Input: part model. Units: mm. Frame: model coordinates. A direction names the side the tool comes from. Give positions to 0.01 mm unless a question says otherwise; leave off trailing zeros. Order: outer loops, then holes, each group sorted by start corner. A loop starts at its lowest first (then second) coordinate and runs counter-clockwise, first axis right, second up. Notation, with made-up numbers: (86, 78) - (98, 78) arc R17 cw to (98, 86) - close; hole circle Ø8 at (4, 22.25). An arc over 180 degrees is marked (long way). Answer in a Markdown table with one row per item. Add a question column.
1. Access query for faces 5 (the face through (0, 213, 101)), 6 (the face through (-1, 79, 100)). Directions: +Z, -Z, +X, -X, +Y, -Y. A direction counts if a zero-diameter tool reaches every point of the face in a straight line with its end or side. Return the directions, or none.
2. Section query D-D on x = -27.5. Return loops of the section in (y, z), and give its area (3 significant figures).
3. Section query A-A on z = 15. Return loops of the section in (x, y), and give its area (3 significant figures).
4. Section query B-B on y = 91.5. Return loops of the section in (x, z), and give its area (3 significant figures).
5. Mould query, pull axis X, two halves, no side actions, for faces 1 (the face through (1, 78, 103)), 2 (the face through (50, 108, 51)), 3 (the face through (-50, 108, 49)), 4 (the face through (-53, 108, 52)). Classes: released by +X, released by -X, zero draft, split by the parting line, or undercut.
6. Section query C-C on z = 56. Return loops of the section in (x, y), and give its area (3 significant figures).
7. Ray query, line 1 (X direction, y = 58, z = 83); line 2 (Z direction, x = -33.5, y = 152). Return the intervals inside material, ascending. Write a range as [from, to].
8. Contact query for a flat-ended pin moving along its axis: pin 1 (1.5 mm diameter, centred on x = -27, y = 22, fed in from -Z). Output: stop coordinate, or through.
Autodesk Inventor part; units mm, degrees
ref_plane "YZ Plane" through (0, 0, 0) normal (1, 0, 0) x (0, 1, 0)
ref_plane "XZ Plane" through (0, 0, 0) normal (0, 1, 0) x (-1, 0, 0)
ref_plane "XY Plane" through (0, 0, 0) normal (0, 0, 1) x (1, 0, 0)
sketch "Sketch2" plane through (0, 0, 0) normal (0, 0, 1) x (1, 0, 0)
  line L0 (53, 53) -> (-53, 53)
  line L1 (-53, 53) -> (-53, -53)
  line L2 (-53, -53) -> (53, -53)
  line L3 (53, -53) -> (53, 53)
  line L4 (53, 53) -> (-53, -53) construction
  line L5 (-53, 53) -> (53, -53) construction
  point P0 (0, 0)
  dimension "d0" = 106
  dimension "d1" = 106
extrude "Extrusion1" add sketch "Sketch2" along normal blind 103
sketch "Sketch3" plane through (-53, -53, 0) normal (0, -1, 0) x (1, 0, 0)
  line L0 (0, 0) -> (106, 0) construction
  line L1 (106, 0) -> (106, 103) construction
  line L2 (0, 103) -> (106, 103) construction
  line L3 (0, 0) -> (0, 103) construction
  line L4 (103, 0) -> (3, 0)
  line L5 (3, 0) -> (3, 100)
  line L6 (3, 100) -> (103, 100)
  line L7 (103, 100) -> (103, 0)
  line L8 (103, 0) -> (3, 100) construction
  line L9 (3, 0) -> (103, 100) construction
  line L10 (53, 127.2) -> (53, -21.2) construction
  point P0 (53, 0)
  point P1 (53, 50)
  point P2 (53, 50)
  point P3 (53, 0)
  dimension "d4" = 3
  dimension "d5" = 3
extrude "Extrusion2" cut sketch "Sketch3" against normal up to surface (106 mm away)
sketch "Sketch4" plane through (53, -53, 0) normal (1, 0, 0) x (0, 0, -1)
  line L0 (0, 0) -> (0, 106) construction
  line L1 (0, 106) -> (-103, 106) construction
  line L2 (-103, 0) -> (-103, 106) construction
  line L3 (0, 0) -> (-103, 0) construction
  line L4 (0, 0) -> (-103, 0)
  line L5 (-103, 0) -> (0, 66)
  line L6 (0, 0) -> (0, 66)
  point P0 (0, 53)
  dimension "d14" = 40
extrude "Extrusion3" cut sketch "Sketch4" against normal up to surface (106 mm away)
sketch "Sketch5" plane through (-53, 53, 103) normal (0, 1, 0) x (1, 0, 0)
  line L0 (3, 3) -> (3, 103) construction
  line L1 (0, 103) -> (0, 0) construction
  line L2 (106, 0) -> (0, 0) construction
  line L3 (106, 103) -> (106, 0) construction
  line L4 (103, 103) -> (103, 3) construction
  line L5 (103, 3) -> (3, 3) construction
  line L6 (103, 103) -> (106, 103)
  line L7 (106, 103) -> (106, 0)
  line L8 (0, 0) -> (0, 103)
  line L9 (3, 103) -> (0, 103)
  line L10 (3, 103) -> (3, 3)
  line L11 (3, 3) -> (103, 3)
  line L12 (103, 3) -> (103, 103)
  line L13 (106, 0) -> (0, 0)
  line L14 (127.2, 103) -> (-21.2, 103) construction
  line L15 (3, 103) -> (0, 103)
  line L16 (106, 103) -> (103, 103)
  point P0 (53, 103)
  point P1 (1.5, 103)
extrude "Extrusion4" add sketch "Sketch5" along normal blind 160
properties part number "P034_Casquette"
Answer:
| question | item | result |
|---|---|---|
| 1 | face 5 | +Z, -Z, +X, -X, +Y |
| 1 | face 6 | -Z, +Y, -Y |
| 2 | outline | (-53, 103) - (-51.08, 100) - (213, 100) - (213, 103) - close |
| 2 | area | 795 mm² |
| 3 | outline | (-53, 3.39) - (-50, 3.39) - (-50, 213) - (-53, 213) - close; (50, 3.39) - (53, 3.39) - (53, 213) - (50, 213) - close |
| 3 | area | 1,260 mm² |
| 4 | outline | (-53, 0) - (-50, 0) - (-50, 100) - (50, 100) - (50, 0) - (53, 0) - (53, 103) - (-53, 103) - close |
| 4 | area | 918 mm² |
| 5 | face 1 | zero draft |
| 5 | face 2 | undercut |
| 5 | face 3 | undercut |
| 5 | face 4 | released by -X |
| 6 | outline | (-53, -22.88) - (-50, -22.88) - (-50, 213) - (-53, 213) - close; (50, -22.88) - (53, -22.88) - (53, 213) - (50, 213) - close |
| 6 | area | 1,420 mm² |
| 7 | line 1 | x = [-53, -50], [50, 53] |
| 7 | line 2 | z = [100, 103] |
| 8 | pin 1 | stops at z = 100 |
